from build123d import *

# Parameters (mm, degrees)
SKETCH1_W                       = 40
SKETCH1_H                       = 40
BOSS_EXTRUDE1_DEPTH             = 4
M3X0_5_TAPPED_HOLE1_D           = 2.5
M3X0_5_TAPPED_HOLE1_CSINK_D     = 3
M3X0_5_TAPPED_HOLE1_CSINK_ANGLE = 90
CUT_EXTRUDE1_DEPTH              = 2
CHAMFER1_SIZE                   = 2
SKETCH7_W                       = 2
SKETCH7_H                       = 4
SKETCH7_W_2                     = 4
SKETCH7_H_2                     = 2
BOSS_EXTRUDE2_DEPTH             = 3
SKETCH12_R                      = 12.88
CUT_EXTRUDE2_DEPTH              = 30.681644159


# Read off the part's stored shape, not the designer's step: M4x0.7 Tapped Hole1, M4x0.7 Tapped Hole2
with BuildPart() as part:
    # Sketch1 → Boss-Extrude1 (new, symmetric)
    with BuildSketch(Plane.XY):
        Rectangle(SKETCH1_W, SKETCH1_H)
    extrude(amount=BOSS_EXTRUDE1_DEPTH, both=True)

    # M3x0.5 Tapped Hole1 (through all)
    with Locations(Plane.XY.offset(4)):
        with Locations((-15, 15), (15, 15), (15, -15), (-15, -15)):
            CounterSinkHole(M3X0_5_TAPPED_HOLE1_D / 2, M3X0_5_TAPPED_HOLE1_CSINK_D / 2, counter_sink_angle=M3X0_5_TAPPED_HOLE1_CSINK_ANGLE)

    # Sketch6 → Cut-Extrude1 (cut)
    with BuildSketch(Plane.XY.offset(4)):
        Polygon((-20, 12), (-12, 12), (-12, 20), (12, 20), (12, 12), (20, 12), (20, -12), (12, -12), (12, -20), (-12, -20), (-12, -12), (-20, -12), align=None)
    extrude(amount=-CUT_EXTRUDE1_DEPTH, mode=Mode.SUBTRACT)

    # Chamfer1
    chamfer1_edges = [part.edges().sort_by_distance(p)[0] for p in [
        (-12, 12, 3),
        (12, 12, 3),
        (12, -12, 3),
        (-12, -12, 3),
    ]]
    chamfer(chamfer1_edges, length=CHAMFER1_SIZE)

    # Sketch7 → Boss-Extrude2 (add)
    with BuildSketch(Plane.XY.offset(2)):
        with Locations((-19, 0)):
            Rectangle(SKETCH7_W, SKETCH7_H)
        with Locations((0, -19)):
            Rectangle(SKETCH7_W_2, SKETCH7_H_2)
    extrude(amount=BOSS_EXTRUDE2_DEPTH)

    # Sketch12 → Cut-Extrude2 (cut, through all)
    with BuildSketch(Plane(origin=(0, 0, -4), x_dir=(-1, 0, 0), z_dir=(0, 0, -1))):
        Circle(SKETCH12_R)
    extrude(amount=-CUT_EXTRUDE2_DEPTH, mode=Mode.SUBTRACT)

    # M4x0.7 Tapped Hole1 outline → M4x0.7 Tapped Hole1 (revolve, cut)
    with BuildSketch(Plane.XY.offset(-1)):
        Polygon((0, 12.773860334), (1.65, 12.773860334), (1.65, 19.65), (2, 20), (0, 20), align=None)
    revolve(axis=Axis((0, 0, -1), (0, 1, 0)), mode=Mode.SUBTRACT)

    # M4x0.7 Tapped Hole2 outline → M4x0.7 Tapped Hole2 (revolve, cut)
    with BuildSketch(Plane.YX.offset(1)):
        Polygon((1.65, -19.65), (1.65, -12.773829877), (0, -12.773829877), (0, -20), (2, -20), align=None)
    revolve(axis=Axis((0, 0, -1), (1, 0, 0)), mode=Mode.SUBTRACT)


solid = part.part
Read the model definition and answer for the solid it produces. Units are mm, in the model's axes. A direction names the side the tool comes from. Coordinates: 2 decimals unless noted, no trailing zeros. Loops run counter-clockwise (first coordinate to the right, second up) from the corner with the lowest first, then second, coordinate; pieces in that order, holes last.
Q1. Each of these flat-tipped pins is pushed along its axis until it touches: pin 1 Ø2.5 at (x, y) = (16.5, -14) entering from +Z; pin 2 Ø1.5 at (x, z) = (-0.5, 4) entering from +Y; pin 3 Ø1.5 at (y, z) = (5.5, 4) entering from -X; pin 4 Ø2.5 at (y, z) = (0.5, 3.5) entering from +X. Where does it stop, or does it pass through?
Q2. Consider probe 1 along X at (y, z) = (15, -1); probe 2 along X at (y, z) = (-15, 3.25); probe 3 along X at (y, z) = (-15, 1.5). Determine where each line is inside the solid, lowest interval first.
Q3. The mould has two halves that part along Y. Classify faces 5 (the face through (-0.3, 20, 1.8)), 6 (the face through (-13, -13, 3)), 7 (the face through (12, 17, 3)): +Y half, -Y half, draft (parallel to the pull), parting line (faces both ways), or undercut.
Q4. The part is cut by section C-C on y = 0. Write down the section's boundary in (x, z).
Q5. The part is cut by section D-D on x = 18.5. Write down the section's boundary in (y, z).
Q6. The part is cut by section A-A on z = 2.75. Give the number of separate pieces and of enclosed holes in the cut face, and give its area (3 significant figures).
Q7. Which of the six approach directions +Z, -Z, +X, -X, +Y, -Y give full straight-line access (tool end or side, diameter ignored) to faces 1 (the face through (-16.164, -0.215, 0.636)), 2 (the face through (-19, 2, 3)), 3 (the face through (-18, 0, 3)), 4 (the face through (-13, 13, 3))?
Q8. The part is cut by section B-B on x = 0. Write down the section's boundary in (y, z), and give its area (3 significant figures).
Results below:
1. pin 1: stops at z = 4
1. pin 2: stops at y = -18
1. pin 3: passes through
1. pin 4: stops at x = -18
2. probe 1: x = -20 to -16.25, -13.75 to -1.65, 1.65 to 13.75, 16.25 to 20
2. probe 2: x = -20 to -16.25, -13.75 to -12, 12 to 13.75, 16.25 to 20
2. probe 3: x = -20 to -16.25, -13.75 to 13.75, 16.25 to 20
3. face 5: +Y half
3. face 6: undercut
3. face 7: draft
4. outline: (-20, -4) - (-12.88, -4) - (-12.88, -2.65) - (-19.65, -2.65) - (-20, -3) - close; (-20, 1) - (-19.65, 0.65) - (-12.88, 0.65) - (-12.88, 2) - (-18, 2) - (-18, 5) - (-20, 5) - close; (12.88, -4) - (20, -4) - (20, 2) - (12.88, 2) - close
5. outline: (-20, -4) - (20, -4) - (20, 4) - (12, 4) - (12, 2) - (-12, 2) - (-12, 4) - (-20, 4) - close
6. separate pieces: 6
6. enclosed holes: 4
6. area: 244 mm2
7. face 1: -X
7. face 2: +Z, +X, -X
7. face 3: +Z, +X
7. face 4: +Z
8. outline: (-20, -4) - (-12.88, -4) - (-12.88, 2) - (-18, 2) - (-18, 5) - (-20, 5) - close; (12.88, -4) - (20, -4) - (20, -3) - (19.65, -2.65) - (12.88, -2.65) - close; (12.88, 0.65) - (19.65, 0.65) - (20, 1) - (20, 2) - (12.88, 2) - close
8. area: 67.8 mm2
